```python
from build123d import *

# Parameters (mm, degrees)
SK_P01_HANGER_W       = 20
SK_P01_HANGER_H       = 8
P01_HANGER_DEPTH      = 29
P02_PIVOTPIN8MM_START = -8.5
SK_P02_PIVOTPIN8MM_R  = 4
P02_PIVOTPIN8MM_DEPTH = 17


with BuildPart() as part:
    # SK_P01_Hanger → P01_Hanger (new body)
    with BuildSketch(Plane(origin=(0, 0, 0), x_dir=(1, 0, 0), z_dir=(0, 1, 0))):
        with Locations((0, 2.5)):
            Rectangle(SK_P01_HANGER_W, SK_P01_HANGER_H)
    extrude(amount=P01_HANGER_DEPTH)

    # SK_P02_Pivotpin8mm → P02_Pivotpin8mm (add)
    with BuildSketch(Plane.XY.offset(P02_PIVOTPIN8MM_START)):
        with Locations((0, 8)):
            Circle(SK_P02_PIVOTPIN8MM_R)
    extrude(amount=P02_PIVOTPIN8MM_DEPTH)


solid = part.part
```
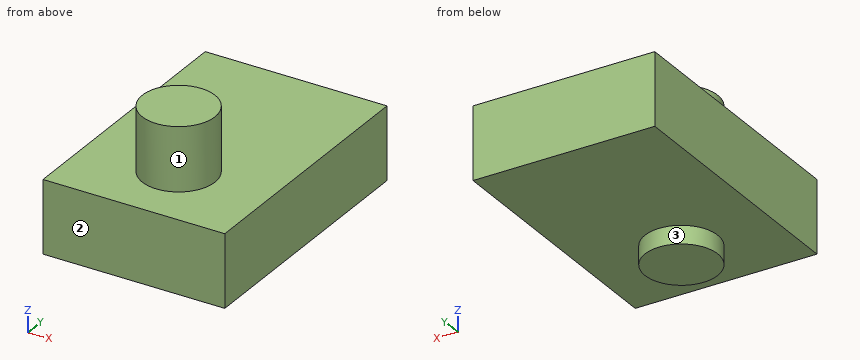
Verification items for the finished model (mm, model axes). Face numbers are marked on the shaded views. A direction names the side the tool comes from. Round coordinates to 2 decimals unless told otherwise and drop trailing zeros. Loops run counter-clockwise (first coordinate to the right, second up) from the corner with the lowest first, then second, coordinate; pieces in that order, holes last. Notation, with made-up numbers: (-14.5, 43) -> (39.5, 43) arc R34 ccw to (39.5, 82) -> close; hole circle Ø1 at (89, 27). An arc over 180 degrees is marked (long way). Answer as a JSON object with one key per item and string values.
Q1. Access from +Z, -Z, +X, -X, +Y, -Y to the whole of each face (thin tool, end or side, straight path). Record for the marked faces 1, 2 and 3.
Data:
{"face 1": "+Z", "face 2": "+Z, -Z, +X, -X, -Y", "face 3": "-Z"}
Q2. Section check D-D (y = 3.25). Record the boundary of the cut face in (x, z), then the cut area to 3 significant figures.
Data:
{"outline": "(-10, -6.5) -> (10, -6.5) -> (10, 1.5) -> (-10, 1.5) -> close", "area": "160 mm2"}
Q3. Section check C-C (x = 7.75). Record the boundary of the cut face in (y, z), then the cut area to 3 significant figures.
Data:
{"outline": "(0, -6.5) -> (29, -6.5) -> (29, 1.5) -> (0, 1.5) -> close", "area": "232 mm2"}
Q4. Section check A-A (y = 8). Record the boundary of the cut face in (x, z), then the cut area to 3 significant figures.
Data:
{"outline": "(-10, -6.5) -> (-4, -6.5) -> (-4, -8.5) -> (4, -8.5) -> (4, -6.5) -> (10, -6.5) -> (10, 1.5) -> (4, 1.5) -> (4, 8.5) -> (-4, 8.5) -> (-4, 1.5) -> (-10, 1.5) -> close", "area": "232 mm2"}
Q5. Go/stop test with a flat-tipped pin: P1, Ø5, axis at x = 1, y = 20, coming from the -Z side. Record where the tip stops, or that it passes through.
Data:
{"P1": "stops at z = -6.5"}
Q6. Scan lines: line 1 (Z direction, x = -6.25, y = 24.5); line 2 (Y direction, x = 0, z = 3); line 3 (X direction, y = 8.25, z = 5.75). Record each from-to range of solid material in increasing order. Write a range as from..to.
Data:
{"line 1": "z = -6.5..1.5", "line 2": "y = 4..12", "line 3": "x = -3.99..3.99"}
Q7. Section check B-B (x = 0). Record the boundary of the cut face in (y, z), then the cut area to 3 significant figures.
Data:
{"outline": "(0, -6.5) -> (4, -6.5) -> (4, -8.5) -> (12, -8.5) -> (12, -6.5) -> (29, -6.5) -> (29, 1.5) -> (12, 1.5) -> (12, 8.5) -> (4, 8.5) -> (4, 1.5) -> (0, 1.5) -> close", "area": "304 mm2"}
